Input: part model. Units: mm. Frame: model coordinates. Give positions to 0.01 mm unless a question says otherwise; leave off trailing zeros. Loops run counter-clockwise (first coordinate to the right, second up) from the corner with the lowest first, then second, coordinate; pieces in that order, holes last.
from build123d import *

# Parameters (mm, degrees)
F0_W          = 88.9
F0_H          = 63.5
F1_DEPTH      = 1
F5_DEPTH      = 25
F7_DEPTH      = 10
F8_R          = 5
F8_R_2        = 6.35
F8_R_3        = 5.08
F8_R_4        = 3.81
F8_R_5        = 3.175
F8_R_6        = 2.54
F8_R_7        = 1.905
F8_R_8        = 1.5875
F8_R_9        = 1.27
F8_R_10       = 0.79375
F8_R_11       = 0.635
F8_R_12       = 4
F8_R_13       = 3
F8_R_14       = 2.5
F8_R_15       = 2
F8_R_16       = 1.5
F8_R_17       = 1.25
F8_R_18       = 1
F8_R_19       = 0.75
F8_R_20       = 0.5
F8_R_21       = 6.82
F9_DEPTH      = 25
F11_DEPTH     = 0.375
F13_DEPTH     = 0.375
F14_T4_DEPTH  = 8.903123749
F14_T10_DEPTH = 8.903123749


# Not quite as in the source:
# - a fillet or chamfer that OpenCascade refuses, or shapes differently, is made with other operations: its cross-section is extruded or revolved along the edge and cut away or added
# - ends of sketch curves that miss each other by under 0.0002 mm in the source are joined


with BuildPart() as f1:
    # F0 (on Top) → F1 (new body)
    with BuildSketch(Plane.XY):
        with Locations((44.45, 31.75)):
            Rectangle(F0_W, F0_H)
    extrude(amount=F1_DEPTH)

    # F4 (on face) → F5 (cut)
    with BuildSketch(Plane.XY.offset(1)):
        with BuildLine():
            Line((78.9, 60.5), (88.9, 60.5))
            Line((88.9, 60.5), (88.9, 62.5))
            Line((88.9, 62.5), (78.9, 62.5))
            ThreePointArc((78.9, 62.5), (79.6071067812, 62.2071067812), (79.9, 61.5))
            ThreePointArc((79.9, 61.5), (79.6071067812, 60.7928932188), (78.9, 60.5))
        make_face()
        with BuildLine():
            ThreePointArc((78.9, 62.5), (77.9, 61.5), (78.9, 60.5))
            Line((78.9, 60.5), (78.9, 62.5))
        make_face()
        with BuildLine():
            Line((78.9, 62.5), (78.9, 60.5))
            ThreePointArc((78.9, 60.5), (79.6071067812, 60.7928932188), (79.9, 61.5))
            ThreePointArc((79.9, 61.5), (79.6071067812, 62.2071067812), (78.9, 62.5))
        make_face()
    extrude(amount=-F5_DEPTH, mode=Mode.SUBTRACT)

    # F6 (on face) → F7 (cut)
    with BuildSketch(Plane.YZ.offset(88.9)):
        with BuildLine():
            add(Edge.make_bspline(
                [(63.5, 0), (63.5, 0.5), (62.5, 0.5)],
                knots=[0, 0, 0, 1.5707963268, 1.5707963268, 1.5707963268], degree=2, weights=[1, 0.7071067812, 1]))
            Line((62.5, 0.5), (62.5, 0))
            Line((62.5, 0), (63.5, 0))
        make_face()
        with BuildLine():
            Line((63.5, 1), (62.5, 1))
            Line((62.5, 1), (62.5, 0.5))
            add(Edge.make_bspline(
                [(62.5, 0.5), (63.5, 0.5), (63.5, 1)],
                knots=[4.7123889804, 4.7123889804, 4.7123889804, 6.2831853072, 6.2831853072, 6.2831853072], degree=2, weights=[1, 0.7071067812, 1]))
        make_face()
    extrude(amount=-F7_DEPTH, mode=Mode.SUBTRACT)

    # F8 (on face) → F9 (cut)
    with BuildSketch(Plane.XY.offset(1)):
        with Locations((74.45, 20)):
            Circle(F8_R)
        with Locations((12.45, 12)):
            Circle(F8_R_2)
        with Locations((27.69, 12)):
            Circle(F8_R_3)
        with Locations((40.39, 12)):
            Circle(F8_R_4)
        with Locations((50.55, 12)):
            Circle(F8_R_5)
        with Locations((58.17, 12)):
            Circle(F8_R_6)
        with Locations((64.52, 12)):
            Circle(F8_R_7)
        with Locations((69.6, 12)):
            Circle(F8_R_8)
        with Locations((73.41, 12)):
            Circle(F8_R_9)
        with Locations((76.585, 12)):
            Circle(F8_R_10)
        with Locations((79.125, 12)):
            Circle(F8_R_11)
        with Locations((59.45, 20)):
            Circle(F8_R_12)
        with Locations((47.45, 20)):
            Circle(F8_R_13)
        with Locations((37.45, 20)):
            Circle(F8_R_14)
        with Locations((29.45, 20)):
            Circle(F8_R_15)
        with Locations((23.45, 20)):
            Circle(F8_R_16)
        with Locations((18.45, 20)):
            Circle(F8_R_17)
        with Locations((14.45, 20)):
            Circle(F8_R_18)
        with Locations((11.45, 20)):
            Circle(F8_R_19)
        with Locations((9.45, 20)):
            Circle(F8_R_20)
        with BuildLine():
            Line((0, 14.9999996647), (2.4641016151, 14.9999996647))
            ThreePointArc((2.4641016151, 14.9999996647), (3.4641016151, 14.9999996647), (3.9641016151, 15.8660250685))
            Line((3.9641016151, 15.8660250685), (4.6961524227, 17.1339742609))
            ThreePointArc((4.6961524227, 17.1339742609), (5.1961524227, 17.9999996647), (4.6961524227, 18.8660250685))
            Line((4.6961524227, 18.8660250685), (3.9641016151, 20.1339742609))
            ThreePointArc((3.9641016151, 20.1339742609), (3.4641016151, 20.9999996647), (2.4641016151, 20.9999996647))
            Line((2.4641016151, 20.9999996647), (0, 20.9999996647))
            Line((0, 20.9999996647), (-1.7320508076, 17.9999996647))
            Line((-1.7320508076, 17.9999996647), (0, 14.9999996647))
        make_face()
        with BuildLine():
            Line((-2.8867513459, 39.0000018477), (0, 34.0000018477))
            Line((0, 34.0000018477), (4.7735026919, 34.0000018477))
            ThreePointArc((4.7735026919, 34.0000018477), (5.2735026919, 33.8660272515), (5.7735026919, 34.0000018477))
            ThreePointArc((5.7735026919, 34.0000018477), (6.1395280957, 34.3660272515), (6.2735026919, 34.8660272515))
            Line((6.2735026919, 34.8660272515), (8.1602540378, 38.133976444))
            ThreePointArc((8.1602540378, 38.133976444), (8.6602540378, 39.0000018477), (8.1602540378, 39.8660272515))
            Line((8.1602540378, 39.8660272515), (6.2735026919, 43.133976444))
            ThreePointArc((6.2735026919, 43.133976444), (5.7735026919, 44.0000018477), (4.7735026919, 44.0000018477))
            Line((4.7735026919, 44.0000018477), (0, 44.0000018477))
            Line((0, 44.0000018477), (-2.8867513459, 39.0000018477))
        make_face()
        with BuildLine():
            Line((0, 23.4999991953), (3.6188021535, 23.4999991953))
            ThreePointArc((3.6188021535, 23.4999991953), (4.6188021535, 23.4999991953), (5.1188021535, 24.3660245991))
            Line((5.1188021535, 24.3660245991), (6.4282032303, 26.6339737916))
            ThreePointArc((6.4282032303, 26.6339737916), (6.9282032303, 27.4999991953), (6.4282032303, 28.3660245991))
            Line((6.4282032303, 28.3660245991), (5.1188021535, 30.6339737916))
            ThreePointArc((5.1188021535, 30.6339737916), (4.6188021535, 31.4999991953), (3.6188021535, 31.4999991953))
            Line((3.6188021535, 31.4999991953), (0, 31.4999991953))
            Line((0, 31.4999991953), (-2.3094010768, 27.4999991953))
            Line((-2.3094010768, 27.4999991953), (0, 23.4999991953))
        make_face()
        with BuildLine():
            Line((0, 46.5000011027), (5.9282032303, 46.5000011027))
            ThreePointArc((5.9282032303, 46.5000011027), (6.9282032303, 46.5000011027), (7.4282032303, 47.3660265065))
            Line((7.4282032303, 47.3660265065), (9.8923048454, 51.6339756989))
            ThreePointArc((9.8923048454, 51.6339756989), (10.3923048454, 52.5000011027), (9.8923048454, 53.3660265065))
            Line((9.8923048454, 53.3660265065), (7.4282032303, 57.6339756989))
            ThreePointArc((7.4282032303, 57.6339756989), (6.9282032303, 58.5000011027), (5.9282032303, 58.5000011027))
            Line((5.9282032303, 58.5000011027), (0, 58.5000011027))
            Line((0, 58.5000011027), (-3.4641016151, 52.5000011027))
            Line((-3.4641016151, 52.5000011027), (0, 46.5000011027))
        make_face()
        with BuildLine():
            ThreePointArc((75.9965413819, 55.4239037183), (69.7064402802, 57.2188103383), (63.4195722631, 55.4126120713))
            ThreePointArc((63.4195722631, 55.4126120713), (62.9586056452, 54.6985726023), (63.2134724878, 53.8877794854))
            Line((63.2134724878, 53.8877794854), (70.453229681, 46.0140204974))
            ThreePointArc((70.453229681, 46.0140204974), (70.6488055759, 45.7004057151), (70.7171076571, 45.3371716473))
            ThreePointArc((70.7171076571, 45.3371716473), (70.080341725, 44.4054737284), (68.9809856332, 44.6603227971))
            Line((68.9809856332, 44.6603227971), (61.74122844, 52.5340817851))
            ThreePointArc((61.74122844, 52.5340817851), (60.9546293112, 52.8559581533), (60.2044919449, 52.4564127647))
            ThreePointArc((60.2044919449, 52.4564127647), (57.8402849867, 44.9987414015), (60.6253238546, 37.6877978778))
            ThreePointArc((60.6253238546, 37.6877978778), (61.2175210997, 37.3466734256), (61.8905196516, 37.4655700956))
            Line((61.8905196516, 37.4655700956), (67.9713955599, 40.9763654382))
            Line((67.9713955599, 40.9763654382), (67.9713955599, 34.4811098251))
            ThreePointArc((67.9713955599, 34.4811098251), (68.2404614442, 33.7986617916), (68.9028661968, 33.4834607253))
            ThreePointArc((68.9028661968, 33.4834607253), (77.6018812733, 36.4487636459), (81.5833352867, 44.7321149393))
            ThreePointArc((81.5833352867, 44.7321149393), (81.3112334204, 45.4700985969), (80.5896132811, 45.7830261909))
            Line((80.5896132811, 45.7830261909), (74.1475280684, 45.7830385939))
            Line((74.1475280684, 45.7830385939), (76.4339684801, 54.3161503788))
            ThreePointArc((76.4339684801, 54.3161503788), (76.3981531684, 54.9422494851), (75.9965413819, 55.4239037183))
        make_face()
        with Locations((69.7171076571, 45.3371716473)):
            Circle(F8_R_20)
        with Locations((23.45, 38.750000298)):
            Circle(F8_R_21)
        with Locations((44.45, 31.75)):
            Circle(F8_R_18)
    extrude(amount=-F9_DEPTH, mode=Mode.SUBTRACT)

    # F10 (on face) → F11 (cut)
    with BuildSketch(Plane.XY.offset(1)):
        Polygon((0, 63.5), (0, 60.5), (4, 63.5), align=None)
    extrude(amount=-F11_DEPTH, mode=Mode.SUBTRACT)

    # F12 (on face) → F13 (cut)
    with BuildSketch(Plane(origin=(0, 0, 0), x_dir=(1, 0, 0), z_dir=(0, 0, -1))):
        Polygon((4, -63.5), (0, -60.5), (0, -63.5), align=None)
    extrude(amount=-F13_DEPTH, mode=Mode.SUBTRACT)

    # F14: fillet of radius 1 on 2 edges, made by hand


with BuildPart() as f14_tool2:
    # F14_s3 → F14_t4 (new body)
    with BuildSketch(Plane(origin=(27.4787505004, 20.6090628753, 0), x_dir=(0, 0, 1), z_dir=(0.8, 0.6, 0))):
        with BuildLine():
            ThreePointArc((1, -48.4), (0.7236121811, -48.7476120479), (0.625, -49.1806247498))
            Line((0.625, -49.1806247498), (0.625, -48.4))
            Line((0.625, -48.4), (1, -48.4))
        make_face()
    extrude(amount=F14_T4_DEPTH)

    split(bisect_by=Plane.YZ, keep=Keep.TOP)

    split(bisect_by=Plane.XZ.offset(-63.5), keep=Keep.TOP)


with BuildPart() as f1_1:
    add(f1.part)

    # F14_t1: union F14_tool2
    add(f14_tool2.part)


with BuildPart() as f14_tool8:
    # F14_s9 → F14_t10 (new body)
    with BuildSketch(Plane(origin=(34.6012494996, 25.9509371247, 0), x_dir=(0, 0, 1), z_dir=(-0.8, -0.6, 0))):
        with BuildLine():
            ThreePointArc((0.375, 49.1806247498), (0.2763878189, 48.7476120479), (0, 48.4))
            Line((0, 48.4), (0.375, 48.4))
            Line((0.375, 48.4), (0.375, 49.1806247498))
        make_face()
    extrude(amount=F14_T10_DEPTH)

    split(bisect_by=Plane.YZ, keep=Keep.TOP)

    split(bisect_by=Plane.XZ.offset(-63.5), keep=Keep.TOP)


with BuildPart() as f1_2:
    add(f1_1.part)

    # F14_t7: union F14_tool8
    add(f14_tool8.part)


solid = f1_2.part
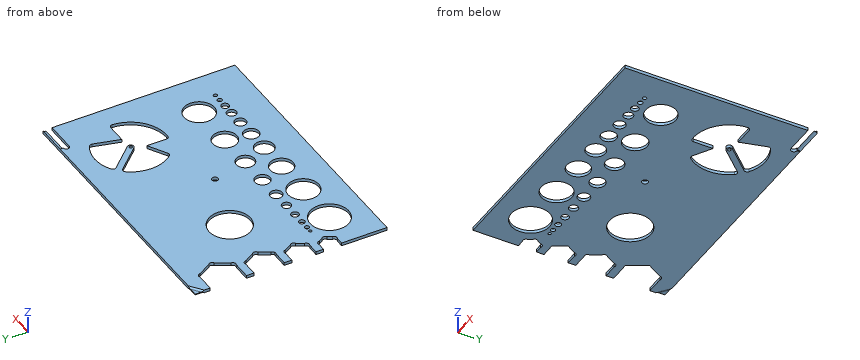
(1) Ray query, probe 1 along X at (y, z) = (50, 0.6); probe 2 along Y at (x, z) = (8, 0.4); probe 3 along X at (y, z) = (44.5, 0.95) (3 decimals). Return the intervals inside material, ascending.
Values follow:
probe 1: x = 8.95 to 58.79, 64.07 to 66.79, 75.28 to 88.9
probe 2: y = 0 to 7.47, 16.53 to 37.86, 40.14 to 48.36, 56.64 to 63.5
probe 3: x = 0 to 19.783, 27.117 to 57.865, 69.17 to 70.264, 81.569 to 88.9
(2) Cut plane A-A (x = 41.5). Return the cut outline in (y, z).
Values follow:
outline: (0, 0) - (8.36, 0) - (8.36, 1) - (0, 1) - close; (15.64, 0) - (63.5, 0) - (63.5, 1) - (15.64, 1) - close
(3) Cut plane B-B (z = 0.8). Count the separate pieces of the cut face and the enclosed holes in it, and give its area (3 significant figures).
Values follow:
separate pieces: 1
enclosed holes: 24
area: 4,320 mm2
(4) Pin query (flat end, axial travel): pin 1 Ø9 at (x, y) = (74.45, 20) entering from +Z. Return the tip coordinate at first contact, or that it passes through.
Values follow:
pin 1: passes through
